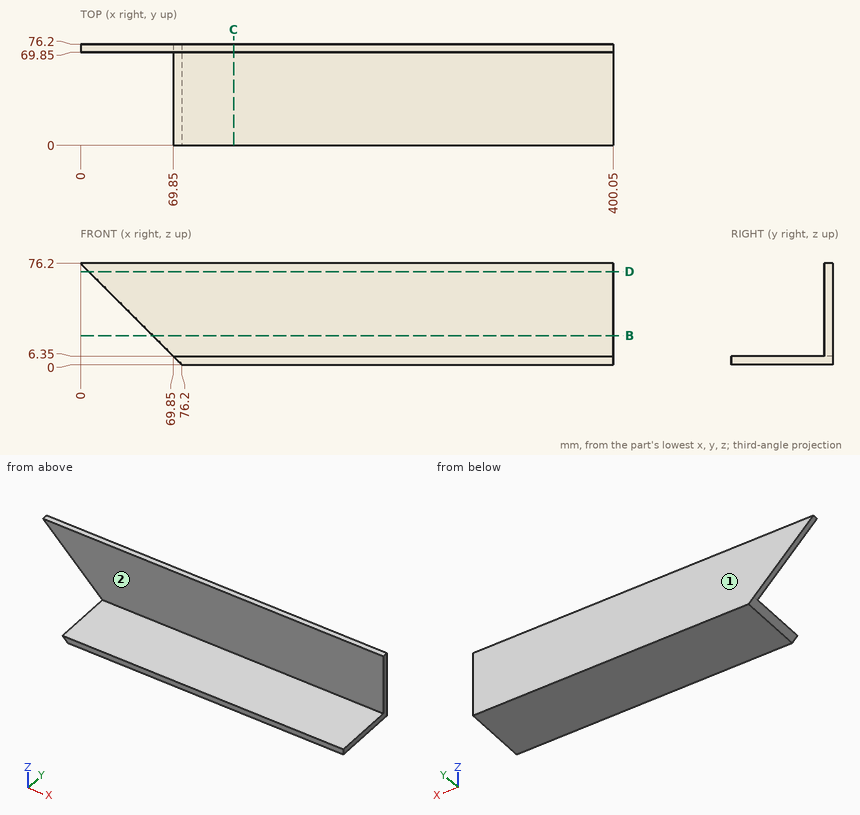
For this review, use the dimensioned drawing (mm, ordinates from the lowest corner) and the shaded views. A direction names the side the tool comes from. Give positions to 0.01 mm unless a question says otherwise; leave off trailing zeros. Write each loop counter-clockwise with the first axis right and the second up, starting at its lowest first coordinate (ties: lowest second). Pieces come first, ordered by that corner, then holes. Notation, with made-up numbers: M 36,49 L 44,49 A12 cw 44,53 Z; hole C 7,-23.75 d7. An arc over 180 degrees is marked long. Write item = value, one per line. Start each with the question number.
Q1. We need section D-D (z = 70). State the section outline as (x, y) points, plus the area to 3 significant figures.
Q2. Clearance check with flat-ended pins moving along their axes: pin 1 (8 mm diameter, centred on x = 332, z = 26, fed in from -Y); pin 2 (4 mm diameter, centred on x = 90.5, y = 28, fed in from +Z). State where each tip first meets the part, or that it passes through.
Q3. For line 1 (Z direction, x = 288.5, y = 63.5); line 2 (Y direction, x = 231, z = 65); line 3 (X direction, y = 21, z = 3.5), list the stretches that pass through material, from the lowest coordinate up.
Q4. Machinability: for the marked faces 1 and 2, which of the approach directions +Z, -Z, +X, -X, +Y, -Y give a long, thin tool a straight path to every point of the face, cutting with its end or side? Answer none if there is none.
Q5. We need section B-B (z = 22). State the section outline as (x, y) points.
Q6. We need section C-C (x = 115). State the section outline as (y, z) points.
Result set:
q1.outline = M 6.2,69.85 L 400.05,69.85 L 400.05,76.2 L 6.2,76.2 Z
q1.area = 2,500 mm2
q2.pin_1 = 69.85
q2.pin_2 = 6.35
q3.line_1 = 0 to 6.35
q3.line_2 = 69.85 to 76.2
q3.line_3 = 72.7 to 400.05
q4.face_1 = +Z, -Z, +X, -X, +Y
q4.face_2 = +Z, +X, -X, -Y
q5.outline = M 54.2,69.85 L 400.05,69.85 L 400.05,76.2 L 54.2,76.2 Z
q6.outline = M 0,0 L 76.2,0 L 76.2,76.2 L 69.85,76.2 L 69.85,6.35 L 0,6.35 Z
